from build123d import *

# Parameters (mm, degrees)
RECPAT_COUNT = 2
RECPAT_ANGLE = 90


with BuildPart() as part:
    # Fillet1: read off the stored shape, not the designer's step
    # Fillet1 outline → Fillet1 (revolve)
    with BuildSketch(Plane.YX):
        with BuildLine():
            Line((1.25, 2.2), (1.25, 8.1))
            Line((1.25, 8.1), (0, 8.1))
            Line((0, 8.1), (0, 0))
            ThreePointArc((0, 0), (1.267435139, 0.206109099), (2.404255321, 0.803195916))
            ThreePointArc((2.404255321, 0.803195916), (2.474733878, 0.88781572), (2.5, 0.99500416))
            Line((2.5, 0.99500416), (2.5, 2.1))
            Line((2.5, 2.1), (1.35, 2.1))
            ThreePointArc((1.35, 2.1), (1.279289322, 2.129289322), (1.25, 2.2))
        make_face()
    revolve(axis=Axis((0, 0, 0), (1, 0, 0)))

    # Sketch3 → Recess section 0
    with BuildSketch(Plane(origin=(0, 0, 0), x_dir=(0, 0, -1), z_dir=(1, 0, 0))):
        with BuildLine():
            Line((0.37, -1.3), (-0.37, -1.3))
            Line((-0.37, -1.3), (-0.37, 1.3))
            Line((-0.37, 1.3), (0.37, 1.3))
            Line((0.37, 1.3), (0.37, -1.3))
        make_face()
    # Sketch4 → Recess section 1
    with BuildSketch(Plane(origin=(1.5, 0, 0), x_dir=(0, 0, -1), z_dir=(1, 0, 0))):
        with BuildLine():
            Line((0.37, -0.552127713), (-0.37, -0.552127713))
            Line((-0.37, -0.552127713), (-0.37, 0.552127713))
            Line((-0.37, 0.552127713), (0.37, 0.552127713))
            Line((0.37, 0.552127713), (0.37, -0.552127713))
        make_face()
    recess = loft(mode=Mode.SUBTRACT)

    # RecPat: Recess ×2 about axis
    recpat_axis = Axis((0, 0, 0), (1, 0, 0))
    for i in range(1, RECPAT_COUNT):
        add(recess.rotate(recpat_axis, i * RECPAT_ANGLE / (RECPAT_COUNT - 1)), mode=Mode.SUBTRACT)

    # RecCorSke → RecessCore (revolve, cut)
    with BuildSketch(Plane.XY, mode=Mode.PRIVATE) as recesscore_sk:
        Polygon((0, 0), (0, 0.660890218), (1.5, 0.556), (1.680655351, 0), align=None)
    revolve(recesscore_sk.sketch.rotate(Axis((-3.175, 0, 0), (1, 0, 0)), 90), axis=Axis((-3.175, 0, 0), (1, 0, 0)), mode=Mode.SUBTRACT)


solid = part.part
The listing builds one solid part. Answer for the finished solid, in the listing's coordinates (mm). Round coordinates to 2 decimals unless told otherwise and drop trailing zeros. Order: outer loops, then holes, each group sorted by start corner. A loop starts at its lowest first (then second) coordinate and runs counter-clockwise, first axis right, second up. Notation, with made-up numbers: (62, -4) -> (96, -4) arc R24 ccw to (96, 21) -> close; hole circle Ø9 at (18.5, 29). An arc over 180 degrees is marked (long way). Write each question's results on one line, items separated by ' | '. Start each with the question number.
Q1. Straight lines are drawn through the part: probe 1 along X at (y, z) = (1.7, -1.1); probe 2 along Y at (x, z) = (1, 1.2); probe 3 along Z at (x, y) = (4, -0.15). For each, find the intervals that lie inside material, in ascending order. Write a range as from..to.
Q2. Find section A-A (x = 6). Determine the outline of the cut face in (y, z).
Q3. The mould has two halves that part along Y. Classify faces 1 (the conical face through (1.67, -0.01, 0.03)), 2 (the cylindrical face through (1.56, -0.54, -2.44)), 3 (the flat face through (8.1, 0, 0)): pulls with the +Y half, pulls with the -Y half, needs draft (parallel to the pull), parting line crosses it, or undercut.
Q4. Each of these flat-tipped pins is pushed along its axis until it touches: pin 1 (2 mm diameter, centred on y = 2, z = 1.5, fed in from +X); pin 2 (2 mm diameter, centred on x = 5, y = 0.5, fed in from +Z). Where does it stop, or does it pass through?
Worked answers:
1) probe 1: x = 0.55..2.1 | probe 2: y = -2.19..2.19 | probe 3: z = -1.24..1.24
2) outline: circle Ø2.5 at (0, 0)
3) face 1: undercut | face 2: parting line crosses it | face 3: needs draft
4) pin 1: stops at x = 2.1 | pin 2: stops at z = 1.25
